Verification items for the finished model (mm, model axes). Face numbers are marked on the shaded views. A direction names the side the tool comes from. Give positions to 0.01 mm unless a question says otherwise; leave off trailing zeros. Write each loop counter-clockwise with the first axis right and the second up, starting at its lowest first coordinate (ties: lowest second). Pieces come first, ordered by that corner, then holes.
from build123d import *

# Parameters (mm, degrees)
F1_DEPTH      = 25.4
F1_DEPTH_BACK = 12.7
F2_T1_DEPTH   = 38.1
F2_T3_DEPTH   = 96.9143148495
F3_W          = 12.7
F3_H          = 12.7
F3_R          = 4.7625
F4_DEPTH      = 25.4
F5_W          = 12.7
F5_H          = 12.7
F6_DEPTH      = 12.7
F6_DEPTH_BACK = 12.7
F7_W          = 63.5
F7_H          = 10.0732017308
F8_DEPTH      = 6.35
F9_SIZE2      = 2.7734531851
F9_SIZE       = 7.62
F9_2_SIZE2    = 2.7734531851
F9_2_SIZE     = 7.62


# Not quite as in the source:
# - a fillet or chamfer that OpenCascade refuses, or shapes differently, is made with other operations: its cross-section is extruded or revolved along the edge and cut away or added


with BuildPart() as f1:
    # F0 (on Front) → F1 (new body, two sides)
    with BuildSketch(Plane.XZ) as f1_sk:
        with BuildLine():
            Line((15.875, 25.4), (-15.875, 25.4))
            ThreePointArc((-15.875, 25.4), (-6.1730633142, 0), (-15.875, -25.4))
            Line((-15.875, -25.4), (15.875, -25.4))
            ThreePointArc((15.875, -25.4), (6.1730633142, 0), (15.875, 25.4))
        make_face()
        with BuildLine():
            ThreePointArc((-9.4926809127, -22.225), (-2.9980633142, 0), (-9.4926809127, 22.225))
            Line((-9.4926809127, 22.225), (9.4926809127, 22.225))
            ThreePointArc((9.4926809127, 22.225), (2.9980633142, 0), (9.4926809127, -22.225))
            Line((9.4926809127, -22.225), (-9.4926809127, -22.225))
        make_face(mode=Mode.SUBTRACT)
    extrude(amount=F1_DEPTH)
    extrude(f1_sk.sketch, amount=-F1_DEPTH_BACK)

    # F2: fillet of radius 6.35 on 8 edges, made by hand

    # F2_s2 → F2_t1 (join)
    with BuildSketch(Plane.XZ.offset(-12.7)):
        with BuildLine():
            ThreePointArc((-0.6282172911, 22.225), (4.5565359978, 19.5411742094), (5.3586201229, 13.7583333333))
            ThreePointArc((5.3586201229, 13.7583333333), (7.1832676704, 18.1100161264), (9.4926809127, 22.225))
            Line((9.4926809127, 22.225), (-0.6282172911, 22.225))
        make_face()
        with BuildLine():
            ThreePointArc((-0.6282172911, -22.225), (4.5565359978, -19.5411742094), (5.3586201229, -13.7583333333))
            ThreePointArc((5.3586201229, -13.7583333333), (7.1832676704, -18.1100161264), (9.4926809127, -22.225))
            Line((9.4926809127, -22.225), (-0.6282172911, -22.225))
        make_face()
        with BuildLine():
            ThreePointArc((0.6282172911, 22.225), (-4.5565359978, 19.5411742094), (-5.3586201229, 13.7583333333))
            ThreePointArc((-5.3586201229, 13.7583333333), (-7.1832676704, 18.1100161264), (-9.4926809127, 22.225))
            Line((-9.4926809127, 22.225), (0.6282172911, 22.225))
        make_face()
        with BuildLine():
            ThreePointArc((-5.3586201229, -13.7583333333), (-4.5565359978, -19.5411742094), (0.6282172911, -22.225))
            Line((0.6282172911, -22.225), (-9.4926809127, -22.225))
            ThreePointArc((-9.4926809127, -22.225), (-7.1832676704, -18.1100161264), (-5.3586201229, -13.7583333333))
        make_face()
    extrude(amount=F2_T1_DEPTH)

    # F2_s4 → F2_t3 (cut)
    with BuildSketch(Plane.XZ.offset(-42.1071574247)):
        with BuildLine():
            ThreePointArc((-4.1121370301, 25.4), (-9.4788665476, 22.4442177723), (-9.8494122136, 16.3285714286))
            ThreePointArc((-9.8494122136, 16.3285714286), (-12.5364180191, 21.0806865498), (-15.875, 25.4))
            Line((-15.875, 25.4), (-4.1121370301, 25.4))
        make_face()
        with BuildLine():
            ThreePointArc((-9.8494122136, -16.3285714286), (-9.4788665476, -22.4442177723), (-4.1121370301, -25.4))
            Line((-4.1121370301, -25.4), (-15.875, -25.4))
            ThreePointArc((-15.875, -25.4), (-12.5364180191, -21.0806865498), (-9.8494122136, -16.3285714286))
        make_face()
        with BuildLine():
            ThreePointArc((4.1121370301, 25.4), (9.4788665476, 22.4442177723), (9.8494122136, 16.3285714286))
            ThreePointArc((9.8494122136, 16.3285714286), (12.5364180191, 21.0806865498), (15.875, 25.4))
            Line((15.875, 25.4), (4.1121370301, 25.4))
        make_face()
        with BuildLine():
            ThreePointArc((9.8494122136, -16.3285714286), (9.4788665476, -22.4442177723), (4.1121370301, -25.4))
            Line((4.1121370301, -25.4), (15.875, -25.4))
            ThreePointArc((15.875, -25.4), (12.5364180191, -21.0806865498), (9.8494122136, -16.3285714286))
        make_face()
    extrude(amount=F2_T3_DEPTH, mode=Mode.SUBTRACT)

    # F3 (on Front) → F4 (join)
    with BuildSketch(Plane.XZ):
        Rectangle(F3_W, F3_H)
        Circle(F3_R, mode=Mode.SUBTRACT)
    extrude(amount=F4_DEPTH)

    # F5 (on Front) → F6 (join, two sides)
    with BuildSketch(Plane.XZ) as f6_sk:
        Rectangle(F5_W, F5_H)
    extrude(amount=-F6_DEPTH)
    extrude(f6_sk.sketch, amount=F6_DEPTH_BACK)

    # F7 (on Right) → F8 (join, symmetric)
    with BuildSketch(Plane.YZ):
        with Locations((30.847759068, 0)):
            Rectangle(F7_W, F7_H)
    extrude(amount=F8_DEPTH, both=True)

    # F9
    f9_edges = [f1.edges().sort_by_distance(p)[0] for p in [
        (6.35, 37.64888, -5.036601),
    ]]
    f9_side = f1.faces().sort_by_distance((6.35, 21.926607, 0))[0]
    chamfer(f9_edges, length=F9_SIZE, length2=F9_SIZE2, reference=f9_side)

    # F9#2
    f9_2_edges = [f1.edges().sort_by_distance(p)[0] for p in [
        (-6.35, 37.64888, -5.036601),
    ]]
    f9_2_side = f1.faces().sort_by_distance((-6.35, 21.926607, 0))[0]
    chamfer(f9_2_edges, length=F9_2_SIZE, length2=F9_2_SIZE2, reference=f9_2_side)


solid = f1.part
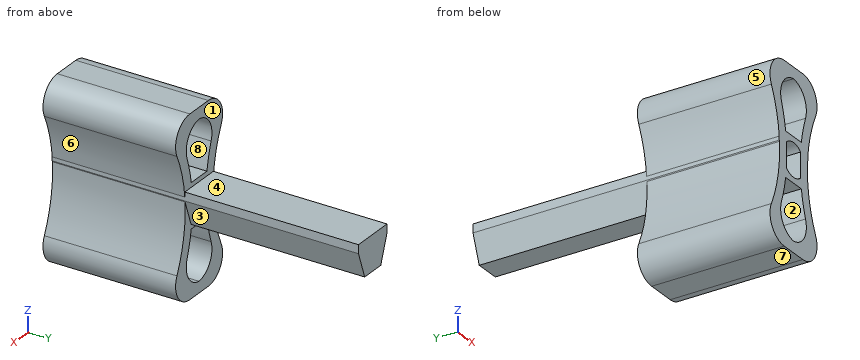
Item 1: Release check for a two-part mould opening along X. For the marked faces 1, 2 and 3 record: released by +X, released by -X, zero draft, split by the parting line, or undercut.
Answer key:
face 1: zero draft
face 2: undercut
face 3: released by +X
Item 2: Sectioned sample at B-B on x = -1. Record the cut outline in (y, z).
Answer key:
outline: (-25.4, -25.4) - (12.7, -25.4) - (12.7, -22.01) - (-25.4, -22.01) - close; (-25.4, -6.35) - (12.7, -6.35) - (12.7, -5.04) - (62.6, -5.04) - (62.6, 5.04) - (12.7, 5.04) - (12.7, 6.35) - (-25.4, 6.35) - (-25.4, 4.66) - (-12.7, 4.66) - (-12.7, -4.66) - (-25.4, -4.66) - close; (-25.4, 22.01) - (12.7, 22.01) - (12.7, 25.4) - (-25.4, 25.4) - close
Item 3: Depth check by flat-ended pin: pin 1 (6.5 mm diameter, centred on x = 1, z = 12.5, fed in from +Y); pin 2 (2.5 mm diameter, centred on y = 34, z = 4, fed in from -X); pin 3 (3 mm diameter, centred on x = -3, y = 34, fed in from +Z); pin 4 (2 mm diameter, centred on y = 2.5, z = 4, fed in from +X). Enter the tip coordinate at first touch or a pass-through.
Answer key:
pin 1: passes through
pin 2: stops at x = -6.35
pin 3: stops at z = 5.04
pin 4: stops at x = 6.5
Item 4: Sectioned sample at A-A on z = 8. Record the cut outline in (x, y).
Answer key:
outline: (-7.02, -25.4) - (-3.78, -25.4) - (-3.78, 12.7) - (-7.02, 12.7) - close; (3.78, -25.4) - (7.02, -25.4) - (7.02, 12.7) - (3.78, 12.7) - close
Item 5: Sectioned sample at C-C on y = 11. Record the cut outline in (x, z) (3 decimals), then the cut area to 3 significant figures.
Answer key:
outline: (-9.849, -16.329) arc R6.35 ccw to (-4.112, -25.4) - (4.112, -25.4) arc R6.35 ccw to (9.849, -16.329) arc R38.1 cw to (6.242, 2.286) - (6.35, 2.583) - (6.35, 3.668) arc R38.1 cw to (9.849, 16.329) arc R6.35 ccw to (4.112, 25.4) - (-4.112, 25.4) arc R6.35 ccw to (-9.849, 16.329) arc R38.1 cw to (-6.35, 3.668) - (-6.35, 2.583) - (-6.242, 2.286) arc R38.1 cw to start; hole (-5.359, -13.758) arc R6.35 ccw to (0, -22.194) arc R6.35 ccw to (5.359, -13.758) arc R41.275 cw to (3.489, -6.35) - (-3.489, -6.35) arc R41.275 cw to start; hole (-5.359, 13.758) arc R41.275 cw to (-3.489, 6.35) - (3.489, 6.35) arc R41.275 cw to (5.359, 13.758) arc R6.35 ccw to (0, 22.194) arc R6.35 ccw to start
area: 539 mm2
Item 6: Set-up check for the marked faces 4, 5, 6, 7 and 8: record each of +Z, -Z, +X, -X, +Y, -Y from which the full face is reachable in a straight line by a thin tool's end or side.
Answer key:
face 4: +Z, +X, -X, +Y
face 5: -X, +Y, -Y
face 6: +X, +Y, -Y
face 7: -Z, +X, -X, +Y, -Y
face 8: +Y, -Y
Item 7: Scan lines: line 1 along Z through (x, y) = (3, -10.5); line 2 along Z through (x, y) = (2.5, -11.5); line 3 along Y through (x, z) = (-5.5, 6). Record each from-to range of solid material in increasing order.
Answer key:
line 1: z = -25.4 to -21.09, -6.35 to 6.35, 21.09 to 25.4
line 2: z = -25.4 to -21.4, -6.35 to 6.35, 21.4 to 25.4
line 3: y = -25.4 to 12.7
Item 8: Sectioned sample at D-D on x = 7.5. Record the cut outline in (y, z).
Answer key:
outline: (-25.4, -24.42) - (12.7, -24.42) - (12.7, -9.97) - (-25.4, -9.97) - close; (-25.4, 9.97) - (12.7, 9.97) - (12.7, 24.42) - (-25.4, 24.42) - close
